Geometry check sheet. Reference: the model listing, model coordinates, mm. A direction names the side the tool comes from. Give positions to 0.01 mm unless a question says otherwise; leave off trailing zeros. Write each loop counter-clockwise with the first axis right and the second up, starting at its lowest first coordinate (ties: lowest second). Pieces come first, ordered by that corner, then holes. Notation, with made-up numbers: (67, -38) - (112, -38) arc R9 cw to (112, -26) - close; hole circle Ø9 at (-16, -33.75). An arc over 180 degrees is marked (long way). One line per question, with ' | ' between items. Start each with the question number.
Q1. Section check A-A on y = 0. Record the boundary of the cut face in (x, z).
Q2. Section check D-D on x = 37.5. Record the boundary of the cut face in (y, z).
Q3. Section check C-C on y = 75. Record the boundary of the cut face in (x, z).
Q4. Section check B-B on z = 10. Record the boundary of the cut face in (x, y).
Q5. Thickness scan on L1, parallel to Y at x = -120, z = 8; L2, parallel to X at y = 74, z = 10; L3, parallel to Y at x = 0, z = 17.75. Record the ranges inside material, lowest first. Write a range as [from, to].
Q6. Release check for a two-part mould opening along Y. For faces 1 (the face through (-107.6, -71.1, 13.3)), 2 (the face through (-148, -2, 13)), 3 (the face through (-2, 123, 13)) record: +Y half, -Y half, draft (parallel to the pull), parting line (faces both ways), or undercut.
Q7. Gauge pin test, flat ends, axial feed: P1, Ø3, axis at x = -107, y = -37.5, coming from the -Z side; P2, Ø21, axis at x = 120, y = -75, coming from the -Z side. Record the tip position at first contact, or that the pin passes through.
Q8. Set-up check for faces 4 (the face through (-2, -123, 13)), 5 (the face through (-20.765, -39.923, 24.535)): record each of +Z, -Z, +X, -X, +Y, -Y from which the full face is reachable in a straight line by a thin tool's end or side.
```python
from build123d import *

# Parameters (mm, degrees)
SKETCH1_W      = 296
SKETCH1_H      = 246
SKETCH1_R      = 13
EXTRUDE1_DEPTH = 27
SKETCH2_R      = 45
EXTRUDE2_DEPTH = 5
SKETCH3_R      = 15
EXTRUDE3_DEPTH = 23


with BuildPart() as part:
    # Sketch1 → Extrude1 (new body)
    with BuildSketch(Plane.XY):
        Rectangle(SKETCH1_W, SKETCH1_H)
        with Locations((-120, 75)):
            Circle(SKETCH1_R, mode=Mode.SUBTRACT)
        with Locations((120, 75)):
            Circle(SKETCH1_R, mode=Mode.SUBTRACT)
        with Locations((120, -75)):
            Circle(SKETCH1_R, mode=Mode.SUBTRACT)
        with Locations((-120, -75)):
            Circle(SKETCH1_R, mode=Mode.SUBTRACT)
    extrude(amount=EXTRUDE1_DEPTH)

    # Sketch2 → Extrude2 (cut)
    with BuildSketch(Plane(origin=(0, 0, 27), x_dir=(-1, 0, 0), z_dir=(0, 0, -1))):
        Circle(SKETCH2_R)
    extrude(amount=EXTRUDE2_DEPTH, mode=Mode.SUBTRACT)

    # Sketch3 → Extrude3 (cut, through all)
    with BuildSketch(Plane.XY.offset(22)):
        Circle(SKETCH3_R)
    extrude(amount=-EXTRUDE3_DEPTH, mode=Mode.SUBTRACT)


solid = part.part
```
Working result:
1) outline: (-148, 0) - (-15, 0) - (-15, 22) - (-45, 22) - (-45, 27) - (-148, 27) - close; (15, 0) - (148, 0) - (148, 27) - (45, 27) - (45, 22) - (15, 22) - close
2) outline: (-123, 0) - (123, 0) - (123, 27) - (24.87, 27) - (24.87, 22) - (-24.87, 22) - (-24.87, 27) - (-123, 27) - close
3) outline: (-148, 0) - (-133, 0) - (-133, 27) - (-148, 27) - close; (-107, 0) - (107, 0) - (107, 27) - (-107, 27) - close; (133, 0) - (148, 0) - (148, 27) - (133, 27) - close
4) outline: (-148, -123) - (148, -123) - (148, 123) - (-148, 123) - close; hole circle Ø26 at (-120, -75); hole circle Ø26 at (-120, 75); hole circle Ø30 at (0, 0); hole circle Ø26 at (120, -75); hole circle Ø26 at (120, 75)
5) L1: y = [-123, -88], [-62, 62], [88, 123] | L2: x = [-148, -132.96], [-107.04, 107.04], [132.96, 148] | L3: y = [-123, -15], [15, 123]
6) face 1: undercut | face 2: draft | face 3: +Y half
7) P1: stops at z = 0 | P2: passes through
8) face 4: +Z, -Z, +X, -X, -Y | face 5: +Z
